```python
from build123d import *

# Parameters (mm, degrees)
SKETCH1_R           = 27
SKETCH1_R_2         = 1.05
BOSS_EXTRUDE1_DEPTH = 3
SKETCH2_R           = 27
SKETCH2_R_2         = 11.65
BOSS_EXTRUDE2_DEPTH = 1.65
SKETCH3_R           = 27
SKETCH3_R_2         = 15.15
BOSS_EXTRUDE3_DEPTH = 5
BOSS_EXTRUDE4_START = 3
SKETCH4_R           = 27
SKETCH4_R_2         = 1.875
BOSS_EXTRUDE4_DEPTH = 3
SKETCH5_W           = 1.5
SKETCH5_H           = 3.970266945
CUT_EXTRUDE1_DEPTH  = 41.224650402
CIRPATTERN1_COUNT   = 8


with BuildPart() as part:
    # Sketch1 → Boss-Extrude1 (new body)
    with BuildSketch(Plane(origin=(0, 0, 0), x_dir=(1, 0, 0), z_dir=(0, 1, 0))):
        with Locations(Location((0, 0, 0), (0, 0, 270))):
            Circle(SKETCH1_R)
        with Locations(Location((0, 7, 0), (0, 0, 270))):
            Circle(SKETCH1_R_2, mode=Mode.SUBTRACT)
        with Locations(Location((0, -7, 0), (0, 0, 270))):
            Circle(SKETCH1_R_2, mode=Mode.SUBTRACT)
    extrude(amount=BOSS_EXTRUDE1_DEPTH)

    # Sketch2 → Boss-Extrude2 (add)
    with BuildSketch(Plane(origin=(0, 3, 0), x_dir=(1, 0, 0), z_dir=(0, 1, 0))):
        with Locations(Location((0, 0, 0), (0, 0, 270))):
            Circle(SKETCH2_R)
        with Locations(Location((0, 0, 0), (0, 0, 270))):
            Circle(SKETCH2_R_2, mode=Mode.SUBTRACT)
    extrude(amount=BOSS_EXTRUDE2_DEPTH)

    # Sketch3 → Boss-Extrude3 (add)
    with BuildSketch(Plane(origin=(0, 4.65, 0), x_dir=(1, 0, 0), z_dir=(0, 1, 0))):
        with Locations(Location((0, 0, 0), (0, 0, 270))):
            Circle(SKETCH3_R)
        with Locations(Location((0, 0, 0), (0, 0, 270))):
            Circle(SKETCH3_R_2, mode=Mode.SUBTRACT)
    extrude(amount=BOSS_EXTRUDE3_DEPTH)

    # Sketch4 → Boss-Extrude4 (add)
    with BuildSketch(Plane.XZ.offset(BOSS_EXTRUDE4_START)):
        with Locations(Location((0, 0, 0), (0, 0, 270))):
            Circle(SKETCH4_R)
        with Locations(Location((0, -7, 0), (0, 0, 270))):
            Circle(SKETCH4_R_2, mode=Mode.SUBTRACT)
        with Locations(Location((0, 7, 0), (0, 0, 270))):
            Circle(SKETCH4_R_2, mode=Mode.SUBTRACT)
    extrude(amount=-BOSS_EXTRUDE4_DEPTH)

    # Sketch5 → Cut-Extrude1 (cut, through all)
    with BuildSketch(Plane(origin=(0, 9.65, 0), x_dir=(1, 0, 0), z_dir=(0, 1, 0))):
        with Locations((0, 25.985133473)):
            Rectangle(SKETCH5_W, SKETCH5_H)
    cut_extrude1 = extrude(amount=-CUT_EXTRUDE1_DEPTH, mode=Mode.SUBTRACT)

    # CirPattern1: Cut-Extrude1 ×8 about axis
    cirpattern1_axis = Axis((0, 0, 0), (0, 1, 0))
    for i in range(1, CIRPATTERN1_COUNT):
        add(cut_extrude1.rotate(cirpattern1_axis, i * 360 / CIRPATTERN1_COUNT), mode=Mode.SUBTRACT)


solid = part.part
```
Can you work these out from the model? Positions are in its coordinate system, mm. A direction names the side the tool comes from. Coordinates: 2 decimals unless noted, no trailing zeros. Loops run counter-clockwise (first coordinate to the right, second up) from the corner with the lowest first, then second, coordinate; pieces in that order, holes last.
1) Imagine slicing it at A-A on y = 1.25. State how many separate pieces and enclosed holes the cut face has, plus the area to 3 significant figures.
2) Thinking about a two-plate mould opening in X: for faces 5 (the flat face through (0, -3, 0)), 6 (the cylindrical face through (-11.37, 3.81, -2.53)), 7 (the flat face through (-1, 0, 8)), 8 (the cylindrical face through (-10.2, 3.2, 25)), which applies, pulls with the +X half, pulls with the -X half, needs draft (parallel to the pull), parting line crosses it, or undercut?
3) I need wall thicknesses on probe 1 along X at (y, z) = (7.55, 0); probe 2 along Y at (x, z) = (8.5, 2); probe 3 along Z at (x, y) = (-4, 5.25). Which ranges of each line are inside material? Lowest first, please.
4) For pin 1 (15 mm diameter, centred on x = 6, z = -2.5, fed in from +Y); pin 2 (4 mm diameter, centred on x = -9.5, y = 1, fed in from -Z); pin 3 (1.5 mm diameter, centred on x = 25.5, y = 3, fed in from -Z), each with a flat end and sliding along its axis, tell me the tip position at first contact or that it passes through.
5) Imagine slicing it at B-B on z = 0. List the corners of the cut face in (x, y) for me, plus the area to 3 significant figures.
6) Which directions (+Z, -Z, +X, -X, +Y, -Y) give clear straight access to the entire face, cutting with the end or side of a thin tool? Please do faces 1 (the flat face through (-24, 3, 0)), 2 (the flat face through (0, 3, 0)), 3 (the cylindrical face through (0.082, -1.521, -5.127)), 4 (the flat face through (18.54, 3.41, 17.48)).
Completed:
1. separate pieces: 1
1. enclosed holes: 2
1. area: 2,250 mm2
2. face 5: needs draft
2. face 6: undercut
2. face 7: undercut
2. face 8: pulls with the -X half
3. probe 1: x = -24 to -15.15, 15.15 to 24
3. probe 2: y = -3 to 3
3. probe 3: z = -26.7 to -14.61, 14.61 to 26.7
4. pin 1: stops at y = 4.65
4. pin 2: stops at z = -25.94
4. pin 3: stops at z = -10.79
5. outline: (-24, -3) - (24, -3) - (24, 9.65) - (15.15, 9.65) - (15.15, 4.65) - (11.65, 4.65) - (11.65, 3) - (-11.65, 3) - (-11.65, 4.65) - (-15.15, 4.65) - (-15.15, 9.65) - (-24, 9.65) - close
5. area: 417 mm2
6. face 1: -X, +Y, -Y
6. face 2: +Y
6. face 3: -Y
6. face 4: +Y, -Y
